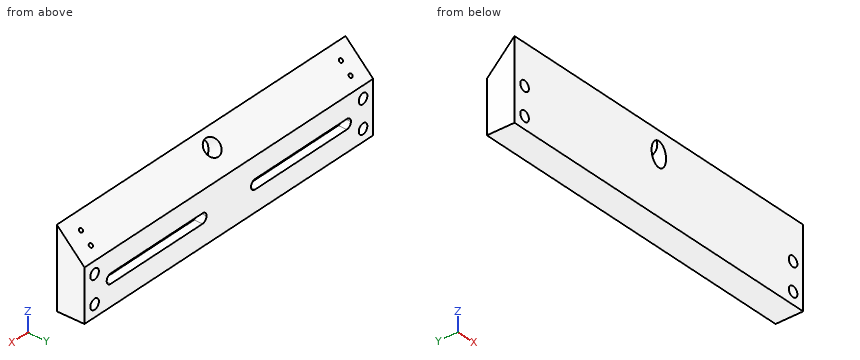
```python
from build123d import *

# Parameters (mm, degrees)
SKETCH1_W           = 254
SKETCH1_H           = 63.5
BOSS_EXTRUDE1_DEPTH = 20.32
CHAMFER1_SIZE       = 25.4
CUT_EXTRUDE1_DEPTH  = 6.35
SKETCH3_R           = 3.7719
CUT_EXTRUDE2_DEPTH  = 133.476280518
SKETCH4_R           = 1.4224
CUT_EXTRUDE3_DEPTH  = 7.366
SKETCH5_R           = 6.35
CUT_EXTRUDE4_DEPTH  = 136.423334215


with BuildPart() as part:
    # Sketch1 → Boss-Extrude1 (new body)
    with BuildSketch(Plane(origin=(0, 0, 0), x_dir=(1, 0, 0), z_dir=(0, 1, 0))):
        Rectangle(SKETCH1_W, SKETCH1_H)
    extrude(amount=BOSS_EXTRUDE1_DEPTH)

    # Chamfer1
    # the kernel refuses this chamfer: 25.4 mm, written as the material it takes off along each edge
    with BuildSketch(Plane(origin=(-192.320747894, 20.32, 31.75), x_dir=(0, -0.9996219169112966, 0.02749587661058647), z_dir=(1, 0, 0))) as chamfer1_piece_1:
        Polygon((CHAMFER1_SIZE * 0.999621916911, CHAMFER1_SIZE * 0.0274958766106), (-CHAMFER1_SIZE * 0.0274958766106, CHAMFER1_SIZE * 0.999621916911), (0, 0), align=None)
    extrude(amount=384.641495789, mode=Mode.SUBTRACT)

    # Sketch2 → Cut-Extrude1 (cut)
    with BuildSketch(Plane(origin=(0, 20.32, 0), x_dir=(1, 0, 0), z_dir=(0, 1, 0))):
        with BuildLine():
            ThreePointArc((-107.442, 12.7), (-106.400471714, 10.185528286), (-103.886, 9.144))
            Line((-103.886, 9.144), (-23.114, 9.144))
            ThreePointArc((-23.114, 9.144), (-20.599528286, 10.185528286), (-19.558, 12.7))
            ThreePointArc((-19.558, 12.7), (-20.599528286, 15.214471714), (-23.114, 16.256))
            Line((-23.114, 16.256), (-103.886, 16.256))
            ThreePointArc((-103.886, 16.256), (-106.400471714, 15.214471714), (-107.442, 12.7))
        make_face()
    cut_extrude1 = extrude(amount=-CUT_EXTRUDE1_DEPTH, mode=Mode.SUBTRACT)

    # Sketch3 → Cut-Extrude2 (cut, through all)
    with BuildSketch(Plane(origin=(0, 20.32, 0), x_dir=(1, 0, 0), z_dir=(0, 1, 0))):
        with Locations(Location((-118.11, 2.54, 0), (0, 0, 270))):
            Circle(SKETCH3_R)
        with Locations(Location((-118.11, 22.86, 0), (0, 0, 90))):
            Circle(SKETCH3_R)
        with Locations(Location((118.11, 2.54, 0), (0, 0, 90))):
            Circle(SKETCH3_R)
        with Locations(Location((118.11, 22.86, 0), (0, 0, 270))):
            Circle(SKETCH3_R)
    extrude(amount=-CUT_EXTRUDE2_DEPTH, mode=Mode.SUBTRACT)

    # Mirror1: Cut-Extrude1 across plane
    add(cut_extrude1.mirror(Plane.ZY), mode=Mode.SUBTRACT)

    # Sketch4 → Cut-Extrude3 (cut)
    with BuildSketch(Plane(origin=(0, 13.335, 13.335), x_dir=(1, 0, 0), z_dir=(0, 0.7071067811865464, 0.7071067811865487))):
        with Locations(Location((-114.3, -8.698537854, 0), (0, 0, 90))):
            Circle(SKETCH4_R)
        with Locations(Location((-114.3, 1.461462146, 0), (0, 0, 270))):
            Circle(SKETCH4_R)
        with Locations(Location((114.3, -8.698537854, 0), (0, 0, 270))):
            Circle(SKETCH4_R)
        with Locations(Location((114.3, 1.461462146, 0), (0, 0, 90))):
            Circle(SKETCH4_R)
    extrude(amount=-CUT_EXTRUDE3_DEPTH, mode=Mode.SUBTRACT)

    # Sketch5 → Cut-Extrude4 (cut, through all)
    with BuildSketch(Plane(origin=(0, 13.335, 13.335), x_dir=(1, 0, 0), z_dir=(0, 0.7071067811865511, 0.707106781186544))):
        with Locations(Location((0, -7.428537854, 0), (0, 0, 270))):
            Circle(SKETCH5_R)
    extrude(amount=-CUT_EXTRUDE4_DEPTH, mode=Mode.SUBTRACT)


solid = part.part
```
Work out the finished part from the listing and answer in its coordinate system (mm). Round coordinates to 2 decimals unless told otherwise and drop trailing zeros. Write each loop counter-clockwise with the first axis right and the second up, starting at its lowest first coordinate (ties: lowest second). Pieces come first, ordered by that corner, then holes.
1) A cutting plane is placed at B-B on x = -118.11. Determine the outline of the cut face in (y, z).
2) Consider probe 1 along X at (y, z) = (6, -22.86); probe 2 along X at (y, z) = (2, -23.5); probe 3 along Z at (x, y) = (-49.5, 16.5). Determine where each line is inside the solid, lowest interval first.
3) A cutting plane is placed at A-A on z = -22.86. Determine the outline of the cut face in (x, y).
4) Flat-ended cylindrical pins translate along their axes: P1, Ø8, axis at x = -29, y = 14, coming from the +Z side; P2, Ø2, axis at x = -64.5, z = 20.5, coming from the +Y side; P3, Ø1.9, axis at x = 45.5, y = 18, coming from the +Z side. Find the tip coordinate at first contact, or state that the pin passes through.
5) A cutting plane is placed at C-C on x = -72. Determine the outline of the cut face in (y, z), and give its area (3 significant figures).
6) A cutting plane is placed at D-D on x = -3. Determine the outline of the cut face in (y, z), and give its area (3 significant figures).
Entries:
1. outline: (0, -31.75) - (20.32, -31.75) - (20.32, -26.63) - (0, -26.63) - close; (0, -19.09) - (20.32, -19.09) - (20.32, -6.31) - (0, -6.31) - close; (0, 1.23) - (20.32, 1.23) - (20.32, 6.35) - (0, 26.67) - close
2. probe 1: x = -127 to -121.88, -114.34 to 114.34, 121.88 to 127
2. probe 2: x = -127 to -121.83, -114.39 to 114.39, 121.83 to 127
2. probe 3: z = -31.75 to -16.26, -9.14 to 10.17
3. outline: (-127, 0) - (-121.88, 0) - (-121.88, 20.32) - (-127, 20.32) - close; (-114.34, 0) - (114.34, 0) - (114.34, 20.32) - (-114.34, 20.32) - close; (121.88, 0) - (127, 0) - (127, 20.32) - (121.88, 20.32) - close
4. P1: stops at z = 16.67
4. P2: stops at y = 7.17
4. P3: stops at z = 9.62
5. outline: (0, -31.75) - (20.32, -31.75) - (20.32, -16.26) - (13.97, -16.26) - (13.97, -9.14) - (20.32, -9.14) - (20.32, 6.35) - (0, 26.67) - close
5. area: 935 mm2
6. outline: (0, -31.75) - (20.32, -31.75) - (20.32, 6.35) - (12.04, 14.63) - (0, 2.59) - close; (0, 18.42) - (4.12, 22.55) - (0, 26.67) - close
6. area: 853 mm2
